Autodesk Inventor part; units mm, degrees
ref_plane "YZ Plane" through (0, 0, 0) normal (1, 0, 0) x (0, 1, 0)
ref_plane "XZ Plane" through (0, 0, 0) normal (0, 1, 0) x (-1, 0, 0)
ref_plane "XY Plane" through (0, 0, 0) normal (0, 0, 1) x (1, 0, 0)
sketch "Sketch1" plane through (0, 0, 0) normal (0, 0, 1) x (1, 0, 0)
  circle A0 centre (0, 0) radius 3.175
  dimension "d0" = 6.35
extrude "Extrusion1" add sketch "Sketch1" along normal blind 12.7
sketch "Sketch2" plane through (0, 0, 12.7) normal (0, 0, 1) x (1, 0, 0)
  point P0 (0, 0)
  point P1 (0, 0)
hole "Hole1" at (0, 0, 12.7) direction (0, 0, -1) diameter 2.6416 depth 10.9728 tip angle 118
sketch "Sketch3" plane through (0, 0, 0) normal (0, 0, -1) x (-1, 0, 0)
  point P0 (0, 0)
  point P1 (0, 0)
hole "Hole2" at (0, 0, 0) at (0, 0, 0) direction (0, 0, 1) diameter 2.6416 depth 10.9728 tip angle 118
properties part number "Standoff"
Geometry check sheet. Reference: the model listing, model coordinates, mm. Give positions to 0.01 mm unless a question says otherwise; leave off trailing zeros. Write each loop counter-clockwise with the first axis right and the second up, starting at its lowest first coordinate (ties: lowest second). Pieces come first, ordered by that corner, then holes.
1) Thickness scan on line 1 (Y direction, x = 0, z = 11.95) (3 decimals); line 2 (X direction, y = 1, z = 2.5); line 3 (Y direction, x = -0.5, z = 7). Record the ranges inside material, lowest first.
Values follow:
line 1: y = -3.175 to -1.321, 1.321 to 3.175
line 2: x = -3.01 to -0.86, 0.86 to 3.01
line 3: y = -3.14 to -1.22, 1.22 to 3.14
2) Cross-section at A-A (y = 0). Record the boundary of the cut face in (x, z) (3 decimals).
Values follow:
outline: (-3.175, 0) - (-1.321, 0) - (-1.321, 12.7) - (-3.175, 12.7) - close; (1.321, 0) - (3.175, 0) - (3.175, 12.7) - (1.321, 12.7) - close
3) Go/stop test with a flat-tipped pin: pin 1 Ø2 at (x, y) = (0, 0) entering from +Z. Record where the tip stops, or that it passes through.
Values follow:
pin 1: passes through
4) Cross-section at C-C (z = 1). Record the boundary of the cut face in (x, y) (3 decimals), plus the area to 3 significant figures.
Values follow:
outline: circle Ø6.35 at (0, 0); hole circle Ø2.642 at (0, 0)
area: 26.2 mm2
5) Cross-section at D-D (x = 2.5). Record the boundary of the cut face in (y, z), plus the area to 3 significant figures.
Values follow:
outline: (-1.96, 0) - (1.96, 0) - (1.96, 12.7) - (-1.96, 12.7) - close
area: 49.7 mm2
6) Cross-section at B-B (x = -0.5). Record the boundary of the cut face in (y, z).
Values follow:
outline: (-3.14, 0) - (-1.22, 0) - (-1.22, 12.7) - (-3.14, 12.7) - close; (1.22, 0) - (3.14, 0) - (3.14, 12.7) - (1.22, 12.7) - close
